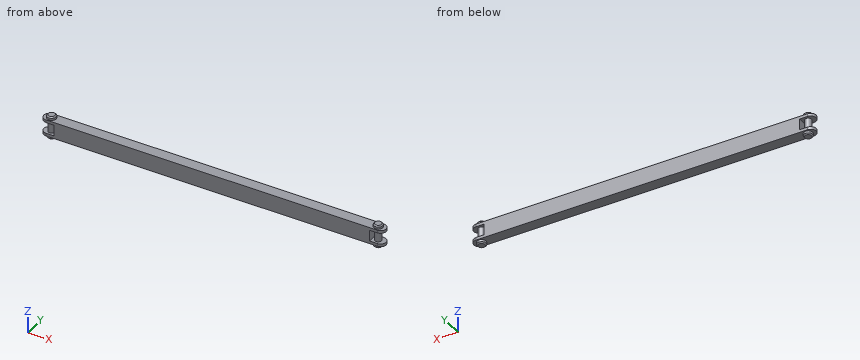
from build123d import *

# Parameters (mm, degrees)
BOSS_EXTRU_1_DEPTH           = 15
ENL_V_MAT_EXTRU_1_REACH      = 312.524
ESQUISSE2_W                  = 12
ESQUISSE2_H                  = 10
BOSS_EXTRU_2_REACH           = 312.413
ESQUISSE3_R                  = 3
ESQUISSE4_R                  = 4
BOSS_EXTRU_3_DEPTH           = 3
CHANFREIN1_SIZE              = 1
CHANFREIN1_OF_SYM_TRIE1_SIZE = 1


with BuildPart() as part:
    # Esquisse1 → Boss.-Extru.1 (new body)
    with BuildSketch(Plane.XY):
        with BuildLine():
            Line((5, 0), (305, 0))
            ThreePointArc((305, 0), (310, 5), (305, 10))
            Line((305, 10), (5, 10))
            ThreePointArc((5, 10), (0, 5), (5, 0))
        make_face()
    extrude(amount=BOSS_EXTRU_1_DEPTH)

    # Esquisse2 → Enlèv. mat.-Extru.1 (cut, up to next)
    with BuildSketch(Plane(origin=(0, 10, 0), x_dir=(1, 0, 0), z_dir=(0, 1, 0)), mode=Mode.PRIVATE) as enl_v_mat_extru_1_sk1:
        with Locations((6, -7.5)):
            Rectangle(ESQUISSE2_W, ESQUISSE2_H)
    enl_v_mat_extru_1_tool1 = extrude(enl_v_mat_extru_1_sk1.sketch, amount=-ENL_V_MAT_EXTRU_1_REACH, mode=Mode.PRIVATE) & part.part
    # Esquisse2 → Enlèv. mat.-Extru.1 (cut, up to next)
    with BuildSketch(Plane(origin=(0, 10, 0), x_dir=(1, 0, 0), z_dir=(0, 1, 0)), mode=Mode.PRIVATE) as enl_v_mat_extru_1_sk2:
        with Locations((304, -7.5)):
            Rectangle(ESQUISSE2_W, ESQUISSE2_H)
    enl_v_mat_extru_1_tool2 = extrude(enl_v_mat_extru_1_sk2.sketch, amount=-ENL_V_MAT_EXTRU_1_REACH, mode=Mode.PRIVATE) & part.part
    add(enl_v_mat_extru_1_tool1.solids().sort_by_distance((6, 10, 7.5))[0], mode=Mode.SUBTRACT)
    add(enl_v_mat_extru_1_tool2.solids().sort_by_distance((304, 10, 7.5))[0], mode=Mode.SUBTRACT)

    # Esquisse3 → Boss.-Extru.2 (add, up to next)
    with BuildSketch(Plane.XY.offset(2.5), mode=Mode.PRIVATE) as boss_extru_2_sk1:
        with Locations(Location((7.054871053, 5, 0), (0, 0, 180))):
            Circle(ESQUISSE3_R)
    boss_extru_2_tool1 = extrude(boss_extru_2_sk1.sketch, amount=BOSS_EXTRU_2_REACH, mode=Mode.PRIVATE) - part.part
    # Esquisse3 → Boss.-Extru.2 (add, up to next)
    with BuildSketch(Plane.XY.offset(2.5), mode=Mode.PRIVATE) as boss_extru_2_sk2:
        with Locations(Location((302.945128947, 5, 0), (0, 0, 180))):
            Circle(ESQUISSE3_R)
    boss_extru_2_tool2 = extrude(boss_extru_2_sk2.sketch, amount=BOSS_EXTRU_2_REACH, mode=Mode.PRIVATE) - part.part
    add(boss_extru_2_tool1.solids().sort_by_distance((7.054871, 5, 2.5))[0])
    add(boss_extru_2_tool2.solids().sort_by_distance((302.945129, 5, 2.5))[0])

    # Esquisse4 → Boss.-Extru.3 (add)
    with BuildSketch(Plane.XY.offset(15)):
        with Locations(Location((7.054871053, 5, 0), (0, 0, 180))):
            Circle(ESQUISSE4_R)
        with Locations(Location((302.945128947, 5, 0), (0, 0, 180))):
            Circle(ESQUISSE4_R)
    boss_extru_3 = extrude(amount=BOSS_EXTRU_3_DEPTH)

    # Chanfrein1
    chanfrein1_edges = [part.edges().sort_by_distance(p)[0] for p in [
        (11.054871053, 5, 18),
        (306.945128947, 5, 18),
    ]]
    chamfer(chanfrein1_edges, length=CHANFREIN1_SIZE)

    # Symétrie1: Boss.-Extru.3 across plane
    add(boss_extru_3.mirror(Plane.XY.offset(7.5)))

    # Chanfrein1 of Symétrie1
    chanfrein1_of_sym_trie1_edges = [part.edges().sort_by_distance(p)[0] for p in [
        (11.054871053, 5, -3),
        (306.945128947, 5, -3),
    ]]
    chamfer(chanfrein1_of_sym_trie1_edges, length=CHANFREIN1_OF_SYM_TRIE1_SIZE)


solid = part.part
CAD build for the part. Positions are in the model's coordinates, mm. Round coordinates to 2 decimals unless told otherwise and drop trailing zeros. Loops run counter-clockwise (first coordinate to the right, second up) from the corner with the lowest first, then second, coordinate; pieces in that order, holes last.
(1) Cut at C-C (x = 288.5). Give the cut face in (y, z).
(2) Drop flat-ended pins along their axis: pin 1 (3 mm diameter, centred on x = 206, y = 5.5, fed in from +Z); pin 2 (4 mm diameter, centred on x = 231.5, y = 2.5, fed in from -Z); pin 3 (3 mm diameter, centred on y = 5, z = 7.5, fed in from +X). Give the stop position or say it passes through.
(3) Cut at B-B (y = 5). State how many separate pieces and enclosed holes the cut face has, plus the area to 3 significant figures.
(4) Cut at A-A (z = 9). Give the cut face in (x, y).
(5) Wall check: line 1 along X through (y, z) = (6.5, 12); line 2 along X through (y, z) = (3.75, 10.5); line 3 along Z through (x, y) = (289.5, 4.25). Give the ranges that are in metal, low to high.
Findings below:
1. outline: (0, 0) - (10, 0) - (10, 15) - (0, 15) - close
2. pin 1: stops at z = 15
2. pin 2: stops at z = 0
2. pin 3: stops at x = 305.95
3. separate pieces: 1
3. enclosed holes: 2
3. area: 4,620 mm2
4. outline: circle Ø6 at (7.05, 5); (12, 0) - (298, 0) - (298, 10) - (12, 10) - close; circle Ø6 at (302.95, 5)
5. line 1: x = 4.46 to 9.65, 12 to 298, 300.35 to 305.54
5. line 2: x = 4.33 to 9.78, 12 to 298, 300.22 to 305.67
5. line 3: z = 0 to 15
